Job drawing, mm, ordinate dimensions from the low corner. One solid piece. A direction names the side the tool comes from. Give positions to 0.01 mm unless a question says otherwise; leave off trailing zeros. Order: outer loops, then holes, each group sorted by start corner. A loop starts at its lowest first (then second) coordinate and runs counter-clockwise, first axis right, second up. Notation, with made-up numbers: (17, -27.75) -> (22, -27.75) arc R26 cw to (22, 7.25) -> close; hole circle Ø11 at (62.25, -15). An arc over 180 degrees is marked (long way). Write item = value, one per line. Start each with the question number.
(1) Saw through at B-B, the plane x = 19. List the corners of the cut face in (y, z).
(2) Saw through at C-C, the plane z = 26. List the corners of the cut face in (x, y).
(3) Flat gauge pin, fed straight in: pin 1 (8 mm diameter, centred on x = 36.5, y = 74, fed in from +Z). Where does the tip first touch, or does it go through?
(4) Saw through at A-A, the plane y = 16.5. List the corners of the cut face in (x, z), then the cut area to 3 significant figures.
(5) Which spindle directions (+Z, -Z, +X, -X, +Y, -Y) get a long thin tool onto all of the face, cutting with end or side? Do the marked faces 1 and 2. Say none if no direction does.
(6) Probe line 1 along Z through (x, y) = (33.5, 54); line 2 along X through (y, z) = (52.5, 53); line 3 along Z through (x, y) = (71, 61.5) (3 decimals). List the from-to ranges inside material, lowest first. Write a range as from..to.
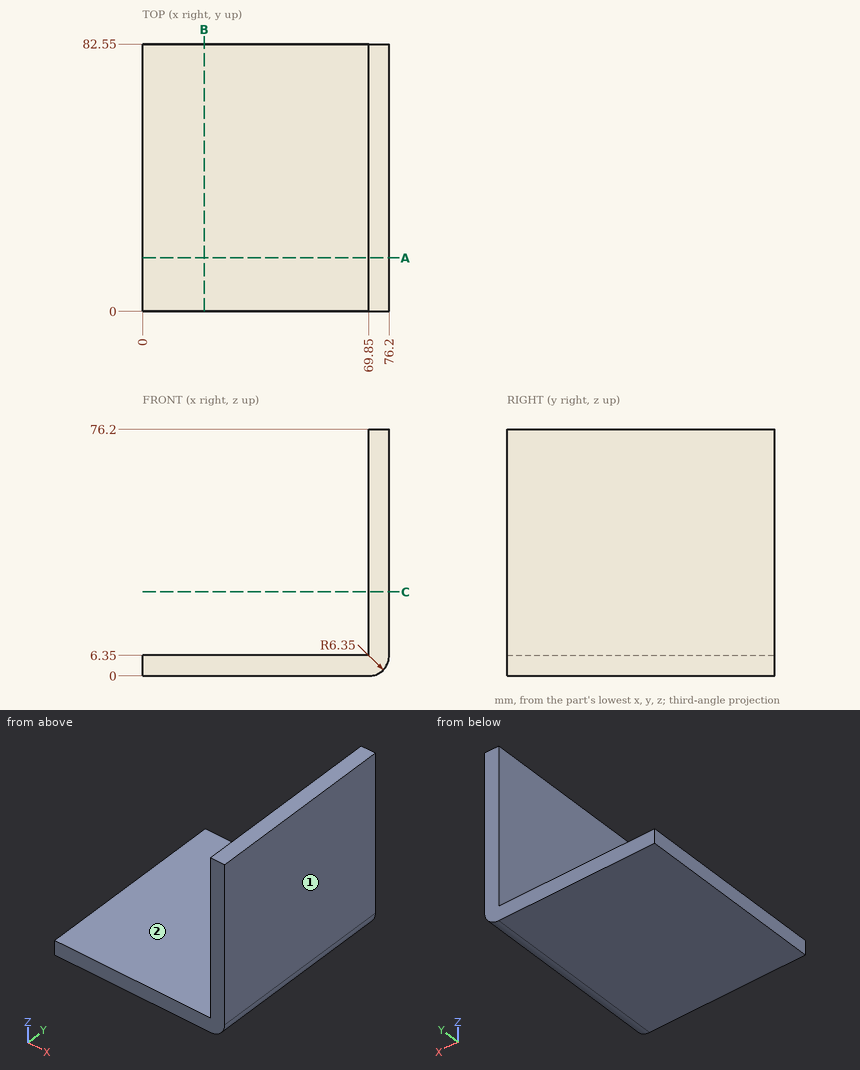
Results list:
q1.outline = (0, 0) -> (82.55, 0) -> (82.55, 6.35) -> (0, 6.35) -> close
q2.outline = (69.85, 0) -> (76.2, 0) -> (76.2, 82.55) -> (69.85, 82.55) -> close
q3.pin_1 = 6.35
q4.outline = (0, 0) -> (69.85, 0) arc R6.35 ccw to (76.2, 6.35) -> (76.2, 76.2) -> (69.85, 76.2) -> (69.85, 6.35) -> (0, 6.35) -> close
q4.area = 919 mm^2
q5.face_1 = +Z, -Z, +X, +Y, -Y
q5.face_2 = +Z, -X, +Y, -Y
q6.line_1 = 0..6.35
q6.line_2 = 69.85..76.2
q6.line_3 = 0.105..76.2
